Source: three-view drawing plus pictorial views. Frame: mm from the lowest corner of the part. Coordinates: 2 decimals unless noted, no trailing zeros. Order: outer loops, then holes, each group sorted by start corner. A loop starts at its lowest first (then second) coordinate and runs counter-clockwise, first axis right, second up. Notation, with made-up numbers: M -40,80 L -12,80 A33 cw -12,111 Z; hole C 30.5,39 d6. An arc over 180 degrees is marked long. One line per question, with ' | ' between items.
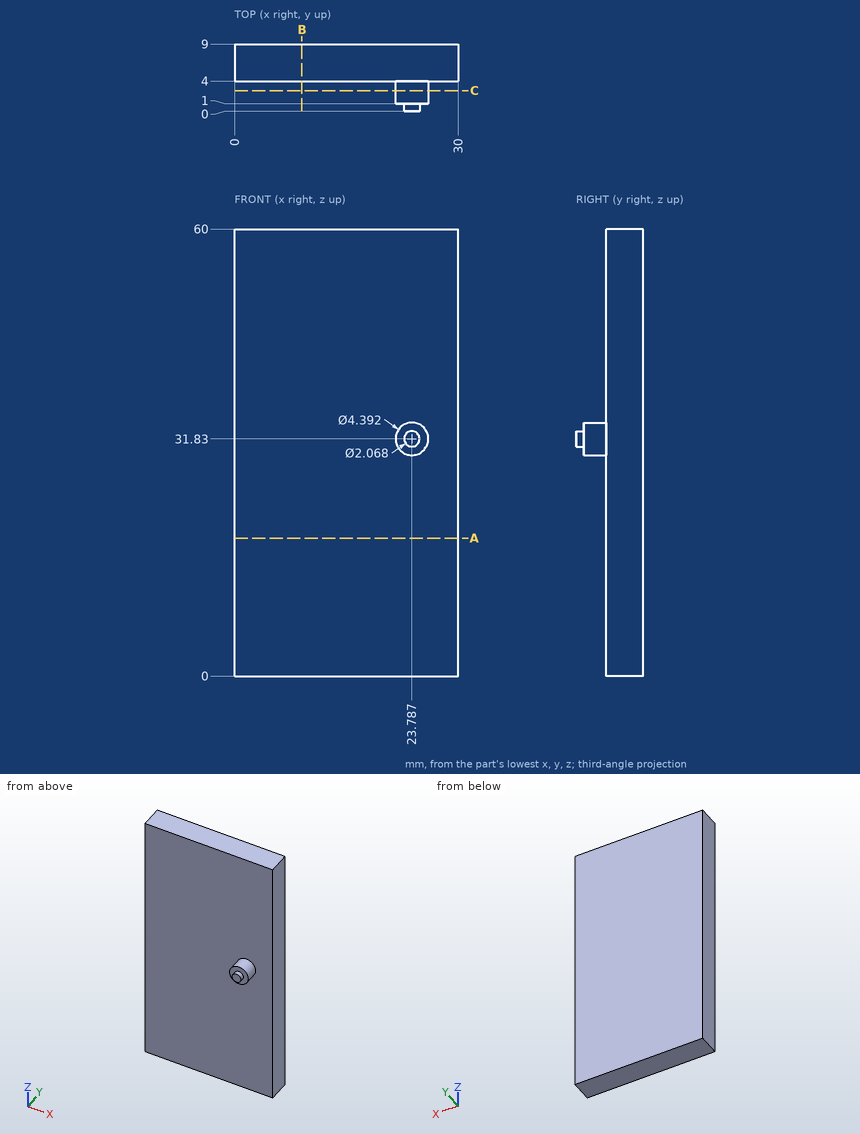
1. Section B-B, the plane x = 9. Output: boundary loops of the cut face in (y, z), and give its area (3 significant figures).
Response values:
outline: M 4,0 L 9,0 L 9,60 L 4,60 Z | area: 300 mm^2
2. Pin query (flat end, axial travel): P1, Ø1, axis at x = 16, y = 8, coming from the -Z side; P2, Ø15, axis at x = 13, z = 41, coming from the -Y side. Return the tip coordinate at first contact, or that it passes through.
Response values:
P1: stops at z = 0 | P2: stops at y = 4
3. Section A-A, the plane z = 18.5. Output: boundary loops of the cut face in (x, y).
Response values:
outline: M 0,4 L 30,4 L 30,9 L 0,9 Z
4. Material intervals for line 1 (Y direction, x = 27, z = 21.5), sorted ascending. Write a range as [from, to].
Response values:
line 1: y = [4, 9]
5. Section C-C, the plane y = 2.75. Output: boundary loops of the cut face in (x, z).
Response values:
outline: C 23.79,31.83 d4.39
